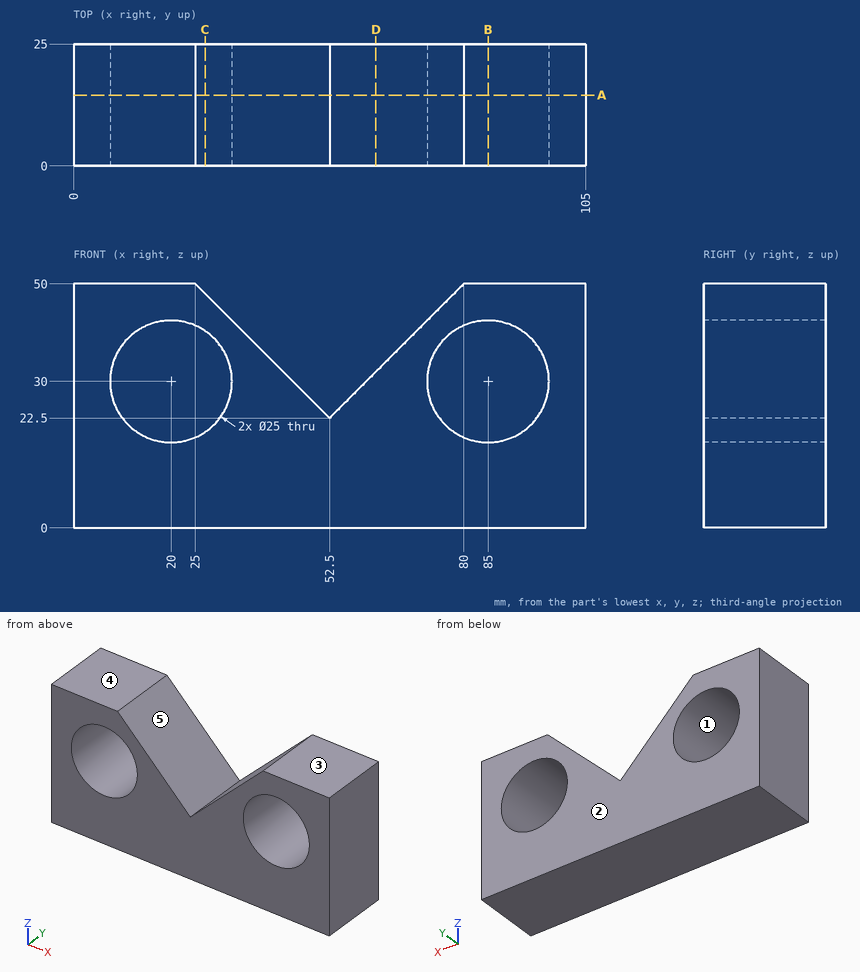
Source: three-view drawing plus pictorial views. Frame: mm from the lowest corner of the part. A direction names the side the tool comes from. Round coordinates to 2 decimals unless told otherwise and drop trailing zeros. Loops run counter-clockwise (first coordinate to the right, second up) from the corner with the lowest first, then second, coordinate; pieces in that order, holes last. Notation, with made-up numbers: M 30,-19.5 L 82,-19.5 A13 ccw 82,-13.5 Z; hole C -33.75,64 d1. An arc over 180 degrees is marked long. Put each result on its own line as item: value. Start each with the question number.
(1) Section query A-A (y = 14.5). Return loops of the section in (x, z).
(2) Material intervals for line 1 along Z through (x, y) = (20, 13.75); line 2 along X through (y, z) = (12.75, 25); line 3 along X through (y, z) = (8.75, 40), sorted ascending. Write a range as [from, to].
(3) Section query B-B (x = 85). Return loops of the section in (y, z).
(4) Section query C-C (x = 27). Return loops of the section in (y, z), then the cut area to 3 significant figures.
(5) Section query D-D (x = 62). Return loops of the section in (y, z).
(6) Draft query along Z for the marked faces 1, 2 and 3. Return one class per face: +Z half, -Z half, draft (parallel to the pull), parting line (faces both ways), or undercut.
(7) Set-up query: the marked faces 4 and 5. Return all of +Z, -Z, +X, -X, +Y, -Y with unobstructed straight access to the full face (end or side cutting, diameter ignored); none if empty.
Findings below:
1. outline: M 0,0 L 105,0 L 105,50 L 80,50 L 52.5,22.5 L 25,50 L 0,50 Z; hole C 20,30 d25; hole C 85,30 d25
2. line 1: z = [0, 17.5], [42.5, 50]
2. line 2: x = [0, 8.54], [31.46, 50], [55, 73.54], [96.46, 105]
2. line 3: x = [0, 12.5], [27.5, 35], [70, 77.5], [92.5, 105]
3. outline: M 0,0 L 25,0 L 25,17.5 L 0,17.5 Z; M 0,42.5 L 25,42.5 L 25,50 L 0,50 Z
4. outline: M 0,0 L 25,0 L 25,19.64 L 0,19.64 Z; M 0,40.36 L 25,40.36 L 25,48 L 0,48 Z
4. area: 682 mm2
5. outline: M 0,0 L 25,0 L 25,32 L 0,32 Z
6. face 1: undercut
6. face 2: draft
6. face 3: +Z half
7. face 4: +Z, +X, -X, +Y, -Y
7. face 5: +Z, +Y, -Y
